from build123d import *

# Parameters (mm, degrees)
SKETCH1_R           = 19.25
SKETCH1_R_2         = 16.25
BOSS_EXTRUDE1_DEPTH = 10
SKETCH2_W           = 70
SKETCH2_H           = 5
BOSS_EXTRUDE2_DEPTH = 10
FILLET1_R           = 10
SKETCH3_R           = 1.75
CUT_EXTRUDE1_DEPTH  = 52.725839771


with BuildPart() as part:
    # Sketch1 → Boss-Extrude1 (new body)
    with BuildSketch(Plane(origin=(0, 0, 0), x_dir=(1, 0, 0), z_dir=(0, 1, 0))):
        with Locations(Location((0, 0, 0), (0, 0, 270))):
            Circle(SKETCH1_R)
        with Locations(Location((0, 0, 0), (0, 0, 270))):
            Circle(SKETCH1_R_2, mode=Mode.SUBTRACT)
    extrude(amount=BOSS_EXTRUDE1_DEPTH)

    # Sketch2 → Boss-Extrude2 (add)
    with BuildSketch(Plane(origin=(0, 0, 0), x_dir=(1, 0, 0), z_dir=(0, 1, 0))):
        with Locations((0, -20)):
            Rectangle(SKETCH2_W, SKETCH2_H)
    extrude(amount=BOSS_EXTRUDE2_DEPTH)

    # Fillet1
    fillet1_edges = [part.edges().sort_by_distance(p)[0] for p in [
        (8.019507466, 5, 17.5),
        (-8.019507466, 5, 17.5),
    ]]
    fillet(fillet1_edges, radius=FILLET1_R)

    # Sketch3 → Cut-Extrude1 (cut, through all)
    with BuildSketch(Plane(origin=(0, 0, 17.5), x_dir=(-1, 0, 0), z_dir=(0, 0, -1))):
        with Locations((30, 5)):
            Circle(SKETCH3_R)
        with Locations((-30, 5)):
            Circle(SKETCH3_R)
    extrude(amount=-CUT_EXTRUDE1_DEPTH, mode=Mode.SUBTRACT)


solid = part.part
Could you check a few things on this model? Use its own coordinates, in mm. A direction names the side the tool comes from. Give positions to 0.01 mm unless a question says otherwise; leave off trailing zeros. Write each loop counter-clockwise with the first axis right and the second up, starting at its lowest first coordinate (ties: lowest second). Pieces come first, ordered by that corner, then holes. Notation, with made-up numbers: (84.5, 16.25) -> (133.5, 16.25) arc R9 ccw to (133.5, 24.25) -> close; hole circle Ø9 at (-35.75, 14.5). An arc over 180 degrees is marked (long way). Answer as a JSON object with one key per item and string values.
Q1. Please list where these lines run through material, in increasing order: L1, parallel to X at y = 5, z = 18.7; L2, parallel to Z at x = -0.5, y = 5.5; L3, parallel to X at y = 4.5, z = 0.
Taken from the geometry:
{"L1": "x = -35 to -31.75, -28.25 to 28.25, 31.75 to 35", "L2": "z = -19.24 to -16.24, 16.24 to 22.5", "L3": "x = -19.25 to -16.25, 16.25 to 19.25"}
Q2. Which directions (+Z, -Z, +X, -X, +Y, -Y) give clear straight access to the entire face, cutting with the end or side of a thin tool? Please do faces 4 (the flat face through (32, 5, 17.5)), 5 (the flat face through (-32, 5, 17.5)), 6 (the flat face through (35, 5, 20)).
Taken from the geometry:
{"face 4": "-Z, +X, +Y, -Y", "face 5": "-Z, -X, +Y, -Y", "face 6": "+Z, -Z, +X, +Y, -Y"}
Q3. We'd pull the mould along Z, two halves only. Please class faces 1 (the flat face through (0, 5, 22.5)), 2 (the cylindrical face through (4.88, 4.93, 15.5)), 3 (the flat face through (-35, 5, 20)): released by +Z, released by -Z, zero draft, split by the parting line, or undercut.
Taken from the geometry:
{"face 1": "released by +Z", "face 2": "undercut", "face 3": "zero draft"}
Q4. Suppose I cut it at B-B on x = 30. Write out the boundary of the cut face in (y, z), then the cut area to 3 significant figures.
Taken from the geometry:
{"outline": "(0, 17.5) -> (3.25, 17.5) -> (3.25, 22.5) -> (0, 22.5) -> close; (6.75, 17.5) -> (10, 17.5) -> (10, 22.5) -> (6.75, 22.5) -> close", "area": "32.5 mm²"}
Q5. Will these pins go through, and if not, where does the flat tip stop? pin 1 Ø5.5 at (x, y) = (31.5, 7) entering from -Z; pin 2 Ø4.5 at (x, y) = (-30, 5) entering from +Z; pin 3 Ø3 at (x, y) = (-15, 8.5) entering from -Z; pin 4 Ø1.5 at (y, z) = (1.5, -5.5) entering from +X.
Taken from the geometry:
{"pin 1": "stops at z = 17.5", "pin 2": "stops at z = 22.5", "pin 3": "stops at z = -13.72", "pin 4": "stops at x = 18.65"}
Q6. Suppose I cut it at A-A on z = 0. Write out the boundary of the cut face in (x, y).
Taken from the geometry:
{"outline": "(-19.25, 0) -> (-16.25, 0) -> (-16.25, 10) -> (-19.25, 10) -> close; (16.25, 0) -> (19.25, 0) -> (19.25, 10) -> (16.25, 10) -> close"}
